Autodesk Inventor part; units mm, degrees
ref_plane "YZ Plane" through (0, 0, 0) normal (1, 0, 0) x (0, 1, 0)
ref_plane "XZ Plane" through (0, 0, 0) normal (0, 1, 0) x (-1, 0, 0)
ref_plane "XY Plane" through (0, 0, 0) normal (0, 0, 1) x (1, 0, 0)
sketch "Sketch5" plane through (0, 0, 0) normal (0, 1, 0) x (-1, 0, 0)
  line L0 (45, 30) -> (-45, 30)
  line L1 (-45, 30) -> (-45, -30)
  line L2 (-45, -30) -> (45, -30)
  line L3 (45, -30) -> (45, 30)
  point P0 (0, 0)
  point P1 (0, 30)
  point P2 (45, 0)
  dimension "d8" = 90
  dimension "d9" = 60
extrude "Extrusion5" add sketch "Sketch5" along normal blind 91.85
sketch "Sketch6" plane through (-45, 0, 30) normal (0, 0, 1) x (1, 0, 0)
  line L0 (0, 0) -> (90, 0)
  line L1 (0, 91.85) -> (90, 91.85)
  line L2 (35, 91.85) -> (55, 91.85)
  line L3 (55, 91.85) -> (55, 65.85)
  line L4 (55, 65.85) -> (35, 65.85)
  line L5 (35, 65.85) -> (35, 91.85)
  point P0 (45, 0)
  point P1 (45, 65.85)
  point P2 (45, 0)
  dimension "d12" = 26
  dimension "d13" = 20
extrude "Extrusion6" add sketch "Sketch6" along normal blind 5
chamfer "Chamfer2" distance 5 angle 45 2 edges at (10, 91.85, 32.5) (-10, 91.85, 32.5)
sketch "Sketch8" plane through (45, 0, -30) normal (0, 0, -1) x (-1, 0, 0)
  line L0 (0, 0) -> (90, 0)
  line L1 (90, 0) -> (90, 91.85)
  line L2 (0, 91.85) -> (90, 91.85)
  line L3 (0, 0) -> (0, 91.85)
  line L4 (20.5, 17) -> (20.5, 91.85)
  line L5 (45, 0) -> (45, 11.253)
  line L6 (45, 91.85) -> (45, 84.4514)
  line L7 (69.5, 91.85) -> (69.5, 17)
  line L8 (77.5, 17) -> (90, 17)
  line L9 (77.5, 17) -> (69.5, 17)
  line L10 (20.5, 17) -> (0, 17)
  point P0 (20.5, 25)
  point P1 (12.5, 17)
  point P2 (69.5, 25)
  dimension "d42" = 90
extrude "Extrusion7" cut sketch "Sketch8" against normal blind 40 contours L3 L2 L4 L10 | L8 L9 L7 L2 L1
sketch "Sketch9" plane through (45, 0, 10) normal (0, 0, -1) x (-1, 0, 0)
  circle A0 centre (10, 77) radius 5
  circle A1 centre (80, 77) radius 5
  line L0 (0, 0) -> (90, 0)
  line L1 (0, 17) -> (0, 91.85)
  circle A2 centre (10, 77) radius 10
  line L2 (0, 91.85) -> (90, 91.85)
  line L3 (45, 91.85) -> (45, 95.8754) construction
  line L4 (20.5, 91.85) -> (20.5, 17) construction
  point P0 (45, 0)
  dimension "d47" = 10
  dimension "d56" = 70
  dimension "d58" = 77
  dimension "d61" = 20
  dimension "d62" = 35
  dimension "d63" = 20.5
hole "Hole2" at (-35, 77, 10) at (35, 77, 10) direction (0, 0, 1) diameter 10.5 end through all
fillet "Fillet3" radius 6 2 edges at (34.75, 17, 10) (-34.75, 17, 10)
sketch "Sketch11" plane through (0, 0, 0) normal (0, -1, 0) x (1, 0, 0)
  line L0 (45, -30) -> (-45, -30)
  circle A0 centre (-35, -8) radius 5.25
  circle A1 centre (35, -8) radius 5.25
  circle A2 centre (-35, -8) radius 10
  line L1 (-24.5, 4) -> (-45, 4)
  point P0 (0, 0)
  dimension "d64" = 70
  dimension "d65" = 10.5
  dimension "d66" = 20
  dimension "d67" = 22
  dimension "d75" = 35
  dimension "d76" = 34
hole "Hole3" at (-35, 0, -8) at (35, 0, -8) direction (0, 1, 0) diameter 10.5 end through all
sketch "Sketch12" plane through (0, 0, 0) normal (0, -1, 0) x (1, 0, 0)
  line L0 (45, 30) -> (40, 30)
  line L1 (45, 25) -> (45, 30)
  line L2 (40, 30) -> (45, 25)
  line L3 (0, 0) -> (-5.6727, 0)
  line L4 (0, 0) -> (0, 4.9012)
  line L5 (45, -30) -> (40, -30)
  line L6 (45, -25) -> (45, -30)
  line L7 (40, -30) -> (45, -25)
  line L8 (-45, 30) -> (-40, 30)
  line L9 (-45, 25) -> (-45, 30)
  line L10 (-40, 30) -> (-45, 25)
  line L11 (-45, -30) -> (-40, -30)
  line L12 (-45, -25) -> (-45, -30)
  line L13 (-40, -30) -> (-45, -25)
  dimension "d80" = 5
  dimension "d81" = 5
extrude "Extrusion8" cut sketch "Sketch12" against normal up to surface (17 mm away) from surface at 0
equation "\"d62\" = 0.5 * d56"
properties part number "BC-10019-A" material "Alumínio 7075"
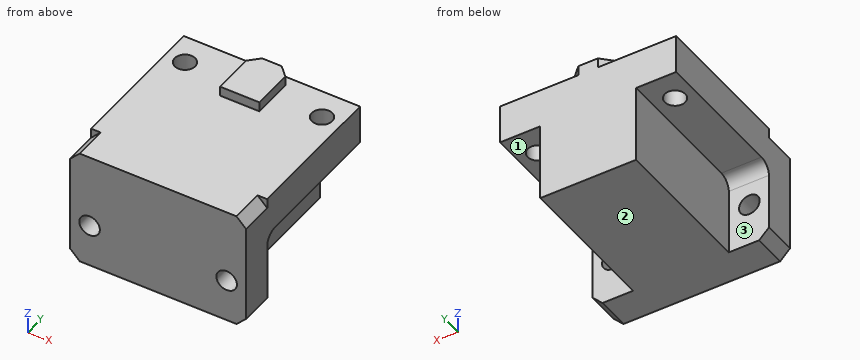
The model under review builds one solid part; all positions refer to its coordinate system, in mm. Face numbers are marked on the shaded views. A direction names the side the tool comes from. Round coordinates to 2 decimals unless told otherwise and drop trailing zeros. Loops run counter-clockwise (first coordinate to the right, second up) from the corner with the lowest first, then second, coordinate; pieces in that order, holes last.
1) Consider section A-A on x = -35. State the section outline as (y, z) points.
Values follow:
outline: (0, -30) - (17, -30) - (17, -13.25) - (0, -13.25) - close; (0, -2.75) - (17, -2.75) - (17, 4) arc R6 cw to (23, 10) - (71.75, 10) - (71.75, 30) - (0, 30) - close; (82.25, 10) - (91.85, 10) - (91.85, 30) - (82.25, 30) - close
2) Wall thickness on line 1 along X through (y, z) = (77, 25.5); line 2 along Y through (x, z) = (-35, 20.5); line 3 along Z through (x, y) = (35, 4): over which ranges is each line inside the solid? List them lowest first.
Values follow:
line 1: x = -45 to -40.25, -29.75 to 29.75, 40.25 to 45
line 2: y = 0 to 71.75, 82.25 to 91.85
line 3: z = -30 to -13.25, -2.75 to 30
3) Clearance check with flat-ended pins moving along their axes: P1, Ø6, axis at x = 40, y = 65.5, coming from the -Z side; P2, Ø4, axis at y = 71.5, z = 32.5, coming from the +X side; P3, Ø6, axis at x = -39.5, z = -7.5, coming from the +Y side. State where each tip first meets the part, or that it passes through.
Values follow:
P1: stops at z = 10
P2: stops at x = 10
P3: stops at y = 17
4) Tool access review of the marked faces 1, 2 and 3: name each direction out of +Z, -Z, +X, -X, +Y, -Y from which nothing blocks a thin tool from reaching the whole face with its end or side.
Values follow:
face 1: -Z, +X, +Y
face 2: -Z, +X, -X, +Y, -Y
face 3: -Z, -X, +Y
5) Consider section D-D on z = 22. State the section outline as (x, y) points, then the cut area to 3 significant figures.
Values follow:
outline: (-45, 0) - (45, 0) - (45, 91.85) - (-45, 91.85) - close; hole circle Ø10.5 at (-35, 77); hole circle Ø10.5 at (35, 77)
area: 8,090 mm2
6) Consider section C-C on z = -8. State the section outline as (x, y) points.
Values follow:
outline: (-45, 0) - (-40.25, 0) - (-40.25, 17) - (-45, 17) - close; (-29.75, 0) - (29.75, 0) - (29.75, 17) - (24.5, 17) - (24.5, 91.85) - (-24.5, 91.85) - (-24.5, 17) - (-29.75, 17) - close; (40.25, 0) - (45, 0) - (45, 17) - (40.25, 17) - close
7) Consider section B-B on y = 77. State the section outline as (x, z) points, then the cut area to 3 significant figures.
Values follow:
outline: (-45, 10) - (-40.25, 10) - (-40.25, 30) - (-45, 30) - close; (-29.75, 10) - (-24.5, 10) - (-24.5, -30) - (24.5, -30) - (24.5, 10) - (29.75, 10) - (29.75, 30) - (10, 30) - (10, 35) - (-10, 35) - (-10, 30) - (-29.75, 30) - close; (40.25, 10) - (45, 10) - (45, 30) - (40.25, 30) - close
area: 3,440 mm2
